The model under review builds one solid part; all positions refer to its coordinate system, in mm. Round coordinates to 2 decimals unless told otherwise and drop trailing zeros. Loops run counter-clockwise (first coordinate to the right, second up) from the corner with the lowest first, then second, coordinate; pieces in that order, holes last. Notation, with made-up numbers: (78, 58) -> (124, 58) arc R26 ccw to (124, 92) -> close; hole circle Ø8 at (54, 46.25). An arc over 180 degrees is marked (long way). Return JSON: item names as keys, results as strings. Group by question number.
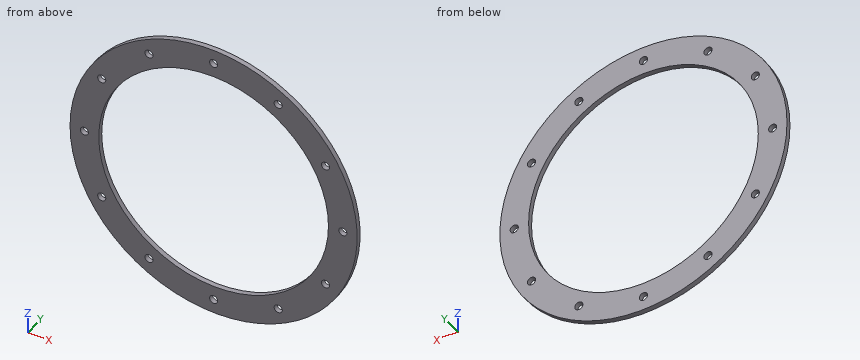
```python
from build123d import *

# Parameters (mm, degrees)
SKETCH1_W                    = 9.525
SKETCH1_H                    = 1.5875
F_36_0_1065_DIAMETER_HOLE1_D = 2.7051
SCREW_PASSTHROUGHS_COUNT     = 12


with BuildPart() as part:
    # Sketch1 → Main (revolve)
    with BuildSketch(Plane.XY):
        with Locations((-42.8625, 0.79375)):
            Rectangle(SKETCH1_W, SKETCH1_H)
    revolve(axis=Axis((0, 55, 0), (0, -1, 0)))

    # #36 (0.1065) Diameter Hole1 (through all)
    with Locations(Plane(origin=(0, 0, 0), x_dir=(-1, 0, 0), z_dir=(0, -1, 0))):
        with Locations((42.8625, 0)):
            f_36_0_1065_diameter_hole1 = Hole(F_36_0_1065_DIAMETER_HOLE1_D / 2)

    # Screw Passthroughs: #36 (0.1065) Diameter Hole1 ×12 about axis
    screw_passthroughs_axis = Axis((0, 0, 0), (0, 1, 0))
    for i in range(1, SCREW_PASSTHROUGHS_COUNT):
        add(f_36_0_1065_diameter_hole1.rotate(screw_passthroughs_axis, i * 360 / SCREW_PASSTHROUGHS_COUNT), mode=Mode.SUBTRACT)


solid = part.part
```
1. We need section D-D, the plane y = 0.3. Give the number of separate pieces and of enclosed holes in the cut face, then the cut area to 3 significant figures.
2. For P1, Ø2, axis at x = -21.43, z = -37.12, coming from the +Y side, flat-tipped, find the tip position at first contact; note if it passes through.
3. We need section B-B, the plane x = 0. Write out the cut boundary in (y, z) (1 decimal).
4. We need section A-A, the plane z = 0. Write out the cut boundary in (x, y) (1 decimal), then the cut area to 3 significant figures.
5. We need section C-C, the plane z = 28. Write out the cut boundary in (x, y).
6. Wall thickness on line 1 (Z direction, x = -0.5, y = 1.45); line 2 (Z direction, x = 4.5, y = 1.45); line 3 (X direction, y = 0.3, z = -8.5): over which ranges is each line inside the solid? List them lowest first.
Check sheet entries:
{
 "1": {"separate pieces": "1", "enclosed holes": "13", "area": "2,500 mm²"},
 "2": {"P1": "passes through"},
 "3": {"outline": "(0, -47.6) -> (1.6, -47.6) -> (1.6, -44.2) -> (0, -44.2) -> close; (0, -41.5) -> (1.6, -41.5) -> (1.6, -38.1) -> (0, -38.1) -> close; (0, 38.1) -> (1.6, 38.1) -> (1.6, 41.5) -> (0, 41.5) -> close; (0, 44.2) -> (1.6, 44.2) -> (1.6, 47.6) -> (0, 47.6) -> close"},
 "4": {"outline": "(-47.6, 0) -> (-44.2, 0) -> (-44.2, 1.6) -> (-47.6, 1.6) -> close; (-41.5, 0) -> (-38.1, 0) -> (-38.1, 1.6) -> (-41.5, 1.6) -> close; (38.1, 0) -> (41.5, 0) -> (41.5, 1.6) -> (38.1, 1.6) -> close; (44.2, 0) -> (47.6, 0) -> (47.6, 1.6) -> (44.2, 1.6) -> close", "area": "21.7 mm²"},
 "5": {"outline": "(-38.52, 0) -> (-25.84, 0) -> (-25.84, 1.59) -> (-38.52, 1.59) -> close; (25.84, 0) -> (38.52, 0) -> (38.52, 1.59) -> (25.84, 1.59) -> close"},
 "6": {"line 1": "z = -47.62 to -44.12, -41.61 to -38.1, 38.1 to 41.61, 44.12 to 47.62", "line 2": "z = -47.41 to -37.83, 37.83 to 47.41", "line 3": "x = -46.86 to -37.14, 37.14 to 46.86"}
}
